Can you work these out from the drawing? Everything is in mm from the part's minimum corner. Give positions to 0.01 mm unless a question says otherwise; leave off trailing zeros. Order: outer loops, then holes, each group sorted by start corner. A loop starts at its lowest first (then second) coordinate and runs counter-clockwise, first axis right, second up. Notation, with made-up numbers: (69, 23.25) - (73, 23.25) arc R15 ccw to (73, 37.25) - close; hole circle Ø4 at (-5, 49.25). An arc over 180 degrees is marked (long way). Write each question's results on one line, items separated by ' | '. Start each with the question number.
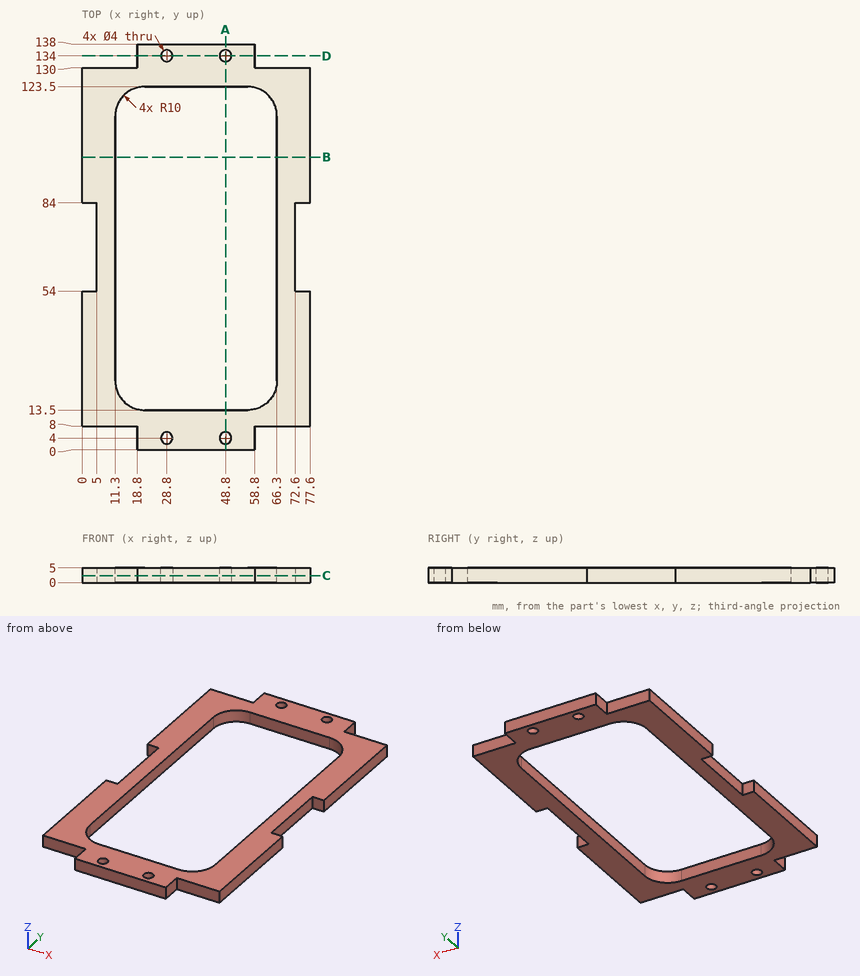
Q1. If I drill on probe 1 along Y at (x, z) = (28.8, 2.6); probe 2 along Y at (x, z) = (43.5, 1); probe 3 along X at (y, z) = (97, 3.85), over which ranges is the centre line in solid material (lowest first)? Write a range as from..to.
Q2. If we section it at C-C (z = 2.3): State how many separate pieces and enclosed holes the cut face has, plus the area to 3 significant figures.
Q3. If we section it at A-A (x = 48.8): Please give me the cut outline in (y, z), plus the area to 3 significant figures.
Q4. If we section it at B-B (y = 99.5): Please give me the cut outline in (x, z), plus the area to 3 significant figures.
Q5. Will these pins go through, and if not, where does the flat tip stop? P1, Ø1.5, axis at y = 3.5, z = 3, coming from the +X side; P2, Ø1.5, axis at y = 2.5, z = 1.5, coming from the -X side; P3, Ø1.5, axis at y = 48.5, z = 2.5, coming from the -X side; P4, Ø1.5, axis at x = 75.5, z = 3.5, coming from the -Y side.
Q6. If we section it at D-D (y = 134): Please give me the cut outline in (x, z), plus the area to 3 significant figures.
Findings below:
1) probe 1: y = 0..2, 6..13.5, 123.5..132, 136..138 | probe 2: y = 0..13.5, 123.5..138 | probe 3: x = 0..11.3, 66.3..77.6
2) separate pieces: 1 | enclosed holes: 5 | area: 3,790 mm2
3) outline: (0, 0) - (2, 0) - (2, 5) - (0, 5) - close; (6, 0) - (13.5, 0) - (13.5, 5) - (6, 5) - close; (123.5, 0) - (132, 0) - (132, 5) - (123.5, 5) - close; (136, 0) - (138, 0) - (138, 5) - (136, 5) - close | area: 100 mm2
4) outline: (0, 0) - (11.3, 0) - (11.3, 5) - (0, 5) - close; (66.3, 0) - (77.6, 0) - (77.6, 5) - (66.3, 5) - close | area: 113 mm2
5) P1: stops at x = 58.8 | P2: stops at x = 18.8 | P3: stops at x = 0 | P4: stops at y = 8
6) outline: (18.8, 0) - (26.8, 0) - (26.8, 5) - (18.8, 5) - close; (30.8, 0) - (46.8, 0) - (46.8, 5) - (30.8, 5) - close; (50.8, 0) - (58.8, 0) - (58.8, 5) - (50.8, 5) - close | area: 160 mm2
